```python
from build123d import *

# Parameters (mm, degrees)
F1_DEPTH = 40
F2_R     = 7.6
F3_DEPTH = 220
F4_DEPTH = 25
F5_SIZE  = 1
F6_R     = 1


with BuildPart() as f1:
    # F0 (on Right) → F1 (new body, symmetric)
    with BuildSketch(Plane.YZ):
        with BuildLine():
            Line((-146.159631235, 0), (0, 0))
            Line((0, 0), (45.9261649855, 0))
            Line((45.9261649855, 0), (103.840368765, 0))
            Line((103.840368765, 0), (103.840368765, 50))
            Line((103.840368765, 50), (-116.159631235, 50))
            Line((-116.159631235, 50), (-116.159631235, 75))
            Line((-116.159631235, 75), (-136.159631235, 75))
            ThreePointArc((-136.159631235, 75), (-143.2306990468, 72.0710678119), (-146.159631235, 65))
            Line((-146.159631235, 65), (-146.159631235, 0))
        make_face()
    extrude(amount=F1_DEPTH, both=True)

    # F2 (on face) → F3 (cut, through all)
    with BuildSketch(Plane(origin=(0, 103.840368765, 0), x_dir=(-1, 0, 0), z_dir=(0, 1, 0))):
        with BuildLine():
            Line((20, 15), (20, 50))
            Line((20, 50), (-20, 50))
            Line((-20, 50), (-20, 15))
            Line((-20, 15), (-15, 15))
            Line((-15, 15), (-9.569428978, 32.9027623113))
            ThreePointArc((-9.569428978, 32.9027623113), (0, 40), (9.569428978, 32.9027623113))
            Line((9.569428978, 32.9027623113), (15, 15))
            Line((15, 15), (20, 15))
        make_face()
        with BuildLine():
            ThreePointArc((10, 30), (9.8917715749, 31.4672610914), (9.569428978, 32.9027623113))
            ThreePointArc((9.569428978, 32.9027623113), (0, 40), (-9.569428978, 32.9027623113))
            ThreePointArc((-9.569428978, 32.9027623113), (-1.4672610914, 20.1082284251), (10, 30))
        make_face()
        with Locations((0, 30)):
            Circle(F2_R, mode=Mode.SUBTRACT)
        with BuildLine():
            Line((-15, 15), (15, 15))
            Line((15, 15), (9.569428978, 32.9027623113))
            ThreePointArc((9.569428978, 32.9027623113), (9.8917715749, 31.4672610914), (10, 30))
            ThreePointArc((10, 30), (-1.4672610914, 20.1082284251), (-9.569428978, 32.9027623113))
            Line((-9.569428978, 32.9027623113), (-15, 15))
        make_face()
        with Locations((0, 30)):
            Circle(F2_R)
    extrude(amount=-F3_DEPTH, mode=Mode.SUBTRACT)

    # F2 (on face) → F4 (join)
    with BuildSketch(Plane(origin=(0, 103.840368765, 0), x_dir=(-1, 0, 0), z_dir=(0, 1, 0))):
        with BuildLine():
            Line((-15, 15), (15, 15))
            Line((15, 15), (9.569428978, 32.9027623113))
            ThreePointArc((9.569428978, 32.9027623113), (9.8917715749, 31.4672610914), (10, 30))
            ThreePointArc((10, 30), (-1.4672610914, 20.1082284251), (-9.569428978, 32.9027623113))
            Line((-9.569428978, 32.9027623113), (-15, 15))
        make_face()
        with BuildLine():
            ThreePointArc((10, 30), (9.8917715749, 31.4672610914), (9.569428978, 32.9027623113))
            ThreePointArc((9.569428978, 32.9027623113), (0, 40), (-9.569428978, 32.9027623113))
            ThreePointArc((-9.569428978, 32.9027623113), (-1.4672610914, 20.1082284251), (10, 30))
        make_face()
        with Locations((0, 30)):
            Circle(F2_R, mode=Mode.SUBTRACT)
    extrude(amount=-F4_DEPTH)

    # F5
    f5_edges = [f1.edges().sort_by_distance(p)[0] for p in [
        (-40, -146.159631, 32.5),
        (-40, -21.159631, 0),
        (-40, 103.840369, 25),
        (-40, -6.159631, 50),
        (-40, -116.159631, 62.5),
        (-40, -126.159631, 75),
        (-40, -143.230699, 72.071068),
        (0, -136.159631, 75),
        (40, -126.159631, 75),
        (0, -116.159631, 75),
        (40, -146.159631, 32.5),
        (40, -21.159631, 0),
        (40, 103.840369, 25),
        (40, -6.159631, 50),
        (40, -116.159631, 62.5),
        (40, -143.230699, 72.071068),
    ]]
    chamfer(f5_edges, length=F5_SIZE)

    # F6
    f6_edges = [f1.edges().sort_by_distance(p)[0] for p in [
        (-12.284714, 103.840369, 23.951381),
        (-15, 91.340369, 15),
        (15, 91.340369, 15),
        (0, 78.840369, 40),
        (-17.5, 103.840369, 15),
        (17.5, 103.840369, 15),
        (12.284714, 103.840369, 23.951381),
        (0, 103.840369, 40),
        (0, 78.840369, 15),
        (-12.284714, 78.840369, 23.951381),
        (12.284714, 78.840369, 23.951381),
    ]]
    fillet(f6_edges, radius=F6_R)


solid = f1.part
```
CAD build for the part. Positions are in the model's coordinates, mm. A direction names the side the tool comes from. Round coordinates to 2 decimals unless told otherwise and drop trailing zeros. Order: outer loops, then holes, each group sorted by start corner. A loop starts at its lowest first (then second) coordinate and runs counter-clockwise, first axis right, second up.
Q1. Slice it at A-A (x = 31.5). Write the cut outline in (y, z).
Q2. Drop a flat-ended pin along its axis: pin 1 (21 mm diameter, centred on x = 33.5, y = 34, fed in from +Z). Give the stop position or say it passes through.
Q3. Wall check: L1, parallel to X at y = -101.5, z = 31; L2, parallel to Y at x = 8, z = 41; L3, parallel to Z at x = 29, y = -113. Give the ranges that are in metal, low to high.
Q4. Slice it at D-D (y = 50). Write the cut outline in (x, z).
Q5. Slice it at C-C (x = 0). Write the cut outline in (y, z), and give its area (3 significant figures).
Q6. Slice it at B-B (z = 46). Write the cut outline in (x, y).
Q7. Two-plate mould, pull along X, no slides. Class faces 1 (the cylindrical face through (11.926, 103.555, 24.099)), 2 (the flat face through (1, -127, 75)), 3 (the conical face through (-39.83, -142.57, 71.56)): pulls with the +X half, pulls with the -X half, needs draft (parallel to the pull), parting line crosses it, or undercut.
Q8. Which spindle directions (+Z, -Z, +X, -X, +Y, -Y) get a long thin tool onto all of the face, cutting with end or side? Do faces 4 (the cylindrical face through (11.9, 79.1, 24.1)), 5 (the flat face through (30, -5, 50)), 6 (the cylindrical face through (-11.85, 103.56, 24.34)). Say none if no direction does.
Results below:
1. outline: (-146.16, 0) - (103.84, 0) - (103.84, 50) - (-116.16, 50) - (-116.16, 74) - (-117.16, 75) - (-136.16, 75) arc R10 ccw to (-146.16, 65) - close
2. pin 1: stops at z = 50
3. L1: x = -40 to -20, 20 to 40
3. L2: y = -146.16 to -116.16
3. L3: z = 0 to 50
4. outline: (-40, 1) - (-39, 0) - (39, 0) - (40, 1) - (40, 49) - (39, 50) - (20, 50) - (20, 15) - (-20, 15) - (-20, 50) - (-39, 50) - (-40, 49) - close
5. outline: (-146.16, 0) - (103.84, 0) - (103.84, 22.4) - (78.84, 22.4) - (78.84, 16) arc R1 cw to (77.84, 15) - (-116.16, 15) - (-116.16, 74) - (-117.16, 75) - (-136.16, 75) arc R10 ccw to (-146.16, 65) - close; (78.84, 37.6) - (103.84, 37.6) - (103.84, 39) arc R1 ccw to (102.84, 40) - (79.84, 40) arc R1 ccw to (78.84, 39) - close
5. area: 5,770 mm2
6. outline: (-40, -145.16) - (-39, -146.16) - (39, -146.16) - (40, -145.16) - (40, 102.84) - (39, 103.84) - (20, 103.84) - (20, -116.16) - (-20, -116.16) - (-20, 103.84) - (-39, 103.84) - (-40, 102.84) - close
7. face 1: undercut
7. face 2: needs draft
7. face 3: pulls with the -X half
8. face 4: +Z
8. face 5: +Z, +X, -X, +Y
8. face 6: +Z, +Y
